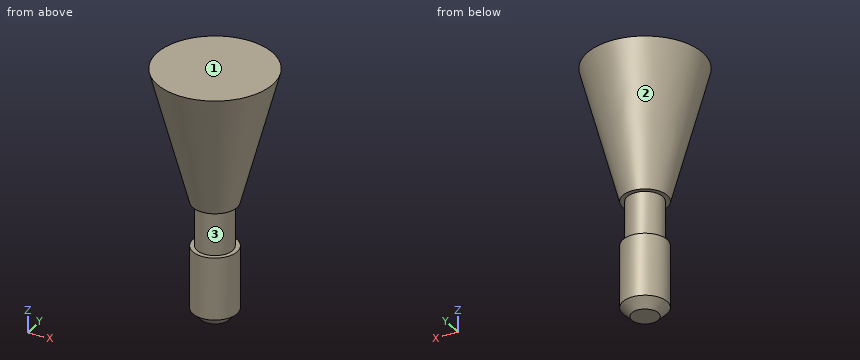
Autodesk Inventor part; units mm, degrees
ref_plane "YZ Plane" through (0, 0, 0) normal (1, 0, 0) x (0, 1, 0)
ref_plane "XZ Plane" through (0, 0, 0) normal (0, 1, 0) x (-1, 0, 0)
ref_plane "XY Plane" through (0, 0, 0) normal (0, 0, 1) x (1, 0, 0)
sketch "Sketch1" plane through (0, 0, 0) normal (0, 0, 1) x (1, 0, 0)
  circle A0 centre (0, 0) radius 3.175
  dimension "d0" = 6.35
extrude "Extrusion1" add sketch "Sketch1" along normal blind 10.16
thread "Thread1"
chamfer "Chamfer1" distance 1.27 angle 45 1 edges at (-3.175, 0, 0)
sketch "Sketch3" plane through (0, 0, 10.16) normal (0, 0, 1) x (1, 0, 0)
  circle A0 centre (0, 0) radius 2.54
  dimension "d11" = 5.08
extrude "Extrusion3" add sketch "Sketch3" along normal blind 6.35
sketch "Sketch4" plane through (0, 0, 16.51) normal (0, 0, 1) x (1, 0, 0)
  circle A0 centre (0, 0) radius 3.175
  dimension "d14" = 6.35
extrude "Extrusion4" add sketch "Sketch4" along normal blind 19.05 draft 15
properties part number "peg-01"
Build history of the part. All positions in model axes, mm. Face numbers are marked on the shaded views. Round coordinates to 2 decimals unless told otherwise and drop trailing zeros. Write each loop counter-clockwise with the first axis right and the second up, starting at its lowest first coordinate (ties: lowest second). Pieces come first, ordered by that corner, then holes.
1) Band-saw the part on A-A, the plane y = 0. List the corners of the cut face in (x, z) (3 decimals).
2) Mould opens along Z. For the marked faces 1, 2 and 3 say: +Z half, -Z half, draft (parallel to the pull), parting line (faces both ways), or undercut.
3) Drill centre lines: probe 1 along X at (y, z) = (-2.5, 26.5); probe 2 along X at (y, z) = (1.5, 27); probe 3 along Y at (x, z) = (-3.5, 31.5). Where is each one in solid material? Low to high.
4) Band-saw the part on C-C, the plane z = 16. List the corners of the cut face in (x, y), and give its area (3 significant figures).
5) Band-saw the part on D-D, the plane z = 31. List the corners of the cut face in (x, y).
6) Pin check, flat tips, straight feed: pin 1 (4 mm diameter, centred on x = -5.5, z = 19.5, fed in from +Y); pin 2 (8 mm diameter, centred on x = -4.5, z = 12, fed in from +Y); pin 3 (1 mm diameter, centred on x = -3, z = 22, fed in from -Y). Stop position of each tip, or through.
Ans:
1. outline: (-8.279, 35.56) - (-3.175, 16.51) - (-2.54, 16.51) - (-2.54, 10.16) - (-3.175, 10.16) - (-3.175, 1.27) - (-1.905, 0) - (1.905, 0) - (3.175, 1.27) - (3.175, 10.16) - (2.54, 10.16) - (2.54, 16.51) - (3.175, 16.51) - (8.279, 35.56) - close
2. face 1: +Z half
2. face 2: -Z half
2. face 3: undercut
3. probe 1: x = -5.29 to 5.29
3. probe 2: x = -5.79 to 5.79
3. probe 3: y = -6.28 to 6.28
4. outline: circle Ø5.08 at (0, 0)
4. area: 20.3 mm2
5. outline: circle Ø14.12 at (0, 0)
6. pin 1: stops at y = 2.05
6. pin 2: stops at y = 3.03
6. pin 3: stops at y = -3.95
